```python
from build123d import *
from OCP.BRepAlgoAPI import BRepAlgoAPI_Cut
from OCP.TopTools import TopTools_ListOfShape

# Parameters (mm, degrees)
SKETCH7_R           = 21.1979112
BOSS_EXTRUDE1_DEPTH = 180.647627
SKETCH12_R          = 20.406966807
BOSS_EXTRUDE6_DEPTH = 50
SHELL1_START        = -50
SHELL1_OUTLINE_R    = 18.406966807
SHELL1_DEPTH        = 100
SHELL1_2_OUTLINE_R  = 19.1979112
SHELL1_2_DEPTH      = 178.6476265
CUT_EXTRUDE1_START  = -22
SKETCH13_R          = 21.1979112
CUT_EXTRUDE1_DEPTH  = 22


with BuildPart() as part:
    # Sketch7 → Boss-Extrude1 (new body)
    with BuildSketch(Plane(origin=(0, 0, 0), x_dir=(1, 0, 0), z_dir=(0, 1, 0))):
        with Locations(Location((0, 0, 0), (0, 0, 270))):
            Circle(SKETCH7_R)
    extrude(amount=BOSS_EXTRUDE1_DEPTH)

    # Sketch12 → Boss-Extrude6 (add, symmetric)
    with BuildSketch(Plane.XY):
        with Locations((0, 116.195122616)):
            Circle(SKETCH12_R)
    extrude(amount=BOSS_EXTRUDE6_DEPTH, both=True)

    # Shell1: read off the stored shape, not the designer's step
    # Shell1 outline → Shell1 (cut)
    with BuildSketch(Plane.XY.offset(SHELL1_START)):
        with Locations((0, 116.195122616)):
            Circle(SHELL1_OUTLINE_R)
    extrude(amount=SHELL1_DEPTH, mode=Mode.SUBTRACT)

    # Shell1 2 outline → Shell1 2 (cut)
    with BuildSketch(Plane(origin=(0, 0, 0), x_dir=(1, 0, 0), z_dir=(0, 1, 0))):
        Circle(SHELL1_2_OUTLINE_R)
    extrude(amount=SHELL1_2_DEPTH, mode=Mode.SUBTRACT)


with BuildPart() as cut_extrude1_tool:
    # Sketch13 → Cut-Extrude1 (new body)
    with BuildSketch(Plane(origin=(0, 180.6476265, 0), x_dir=(1, 0, 0), z_dir=(0, 1, 0)).offset(CUT_EXTRUDE1_START)):
        with Locations(Location((0, 0, 0), (0, 0, 270))):
            Circle(SKETCH13_R)
    extrude(amount=CUT_EXTRUDE1_DEPTH)


with BuildPart() as part_1:
    add(part.part)

    # Cut-Extrude1: cut by cut_extrude1_tool, with a tolerance
    cut_extrude1_stock = TopTools_ListOfShape()
    cut_extrude1_stock.Append(part_1.part.wrapped)
    cut_extrude1_tools = TopTools_ListOfShape()
    cut_extrude1_tools.Append(cut_extrude1_tool.part.wrapped)
    cut_extrude1_cut = BRepAlgoAPI_Cut()
    cut_extrude1_cut.SetArguments(cut_extrude1_stock)
    cut_extrude1_cut.SetTools(cut_extrude1_tools)
    cut_extrude1_cut.SetFuzzyValue(0.00001)
    cut_extrude1_cut.Build()
    add(Compound.cast(cut_extrude1_cut.Shape()).solids(), mode=Mode.REPLACE)


solid = part_1.part
```
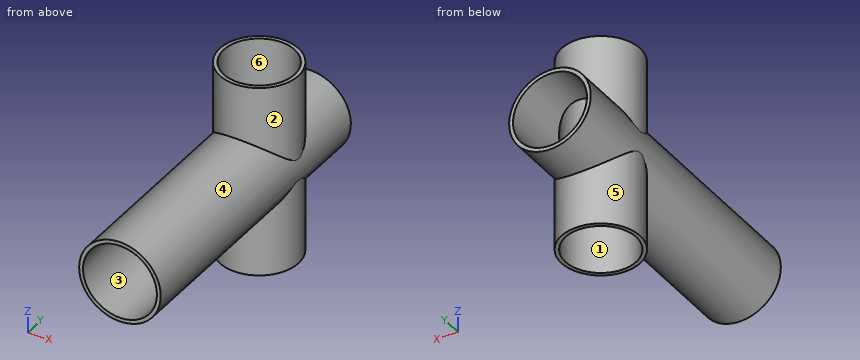
Input: part model. Units: mm. Frame: model coordinates. Face numbers are marked on the shaded views. A direction names the side the tool comes from. Round coordinates to 2 decimals unless told otherwise and drop trailing zeros. Loops run counter-clockwise (first coordinate to the right, second up) from the corner with the lowest first, then second, coordinate; pieces in that order, holes last. Notation, with made-up numbers: (-23.75, -24.5) -> (-0.75, -24.5) arc R29 cw to (-0.75, 12.5) -> close; hole circle Ø8 at (39.5, 33.25). An arc over 180 degrees is marked (long way). Use one line per item in the form item = value. Start each with the question number.
Item 1: Set-up query: the marked faces 4, 5 and 6. Return all of +Z, -Z, +X, -X, +Y, -Y with unobstructed straight access to the full face (end or side cutting, diameter ignored); none if empty.
Item 2: Section query C-C on y = 110.5. Return the cut outline in (x, z), then the cut area to 3 significant figures.
Item 3: Section query A-A on z = 0. Return the cut outline in (x, y).
Item 4: Mould query, pull axis Y, two halves, no side actions, for the marked faces 1, 2 and 3. Classes: pulls with the +Y half, pulls with the -Y half, needs draft (parallel to the pull), parting line crosses it, or undercut.
Item 5: Contact query for flat-ended pins moving along their axis: pin 1 Ø2 at (y, z) = (19.5, -20.5) entering from -X; pin 2 Ø2 at (x, z) = (1.5, -19) entering from -Y; pin 3 Ø1 at (x, y) = (11.5, 27.5) entering from -Z; pin 4 Ø4 at (x, z) = (0.5, 32.5) entering from +Y. Output: stop coordinate, or through.
Item 6: Section query B-B on x = 0. Return the cut outline in (y, z).
Item 7: Material intervals for L1, parallel to X at y = 121, z = 0; L2, parallel to Y at x = 0, z = -27, sorted ascending. Write a range as from..to.
Item 8: Section query D-D on x = -13.5. Return the cut outline in (y, z).
Ans:
q1.face_4 = none
q1.face_5 = -Z
q1.face_6 = +Z, -Z
q2.outline = (-19.6, -50) -> (-17.5, -50) -> (-17.5, -7.89) arc R19.2 cw to (-17.5, 7.89) -> (-17.5, 50) -> (-19.6, 50) -> (-19.6, 8.08) arc R21.2 ccw to (-19.6, -8.08) -> close; (17.5, -50) -> (19.6, -50) -> (19.6, -8.08) arc R21.2 ccw to (19.6, 8.08) -> (19.6, 50) -> (17.5, 50) -> (17.5, 7.89) arc R19.2 cw to (17.5, -7.89) -> close
q2.area = 417 mm^2
q3.outline = (-21.2, 0) -> (-19.2, 0) -> (-19.2, 158.65) -> (-21.2, 158.65) -> close; (19.2, 0) -> (21.2, 0) -> (21.2, 158.65) -> (19.2, 158.65) -> close
q4.face_1 = undercut
q4.face_2 = parting line crosses it
q4.face_3 = needs draft
q5.pin_1 = -8.31
q5.pin_2 = 0
q5.pin_3 = -18.12
q5.pin_4 = 136.6
q6.outline = (0, -21.2) -> (95.79, -21.2) -> (95.79, -50) -> (97.79, -50) -> (97.79, -19.2) -> (0, -19.2) -> close; (0, 19.2) -> (97.79, 19.2) -> (97.79, 50) -> (95.79, 50) -> (95.79, 21.2) -> (0, 21.2) -> close; (134.6, -50) -> (136.6, -50) -> (136.6, -21.2) -> (158.65, -21.2) -> (158.65, -19.2) -> (134.6, -19.2) -> close; (134.6, 19.2) -> (158.65, 19.2) -> (158.65, 21.2) -> (136.6, 21.2) -> (136.6, 50) -> (134.6, 50) -> close
q7.L1 = -21.2..-19.2, 19.2..21.2
q7.L2 = 95.79..97.79, 134.6..136.6
q8.outline = (0, -16.34) -> (100.89, -16.34) -> (100.89, -50) -> (103.68, -50) -> (103.68, -13.65) -> (0, -13.65) -> close; (0, 13.65) -> (103.68, 13.65) -> (103.68, 50) -> (100.89, 50) -> (100.89, 16.34) -> (0, 16.34) -> close; (128.71, -50) -> (131.5, -50) -> (131.5, -16.34) -> (158.65, -16.34) -> (158.65, -13.65) -> (128.71, -13.65) -> close; (128.71, 13.65) -> (158.65, 13.65) -> (158.65, 16.34) -> (131.5, 16.34) -> (131.5, 50) -> (128.71, 50) -> close
